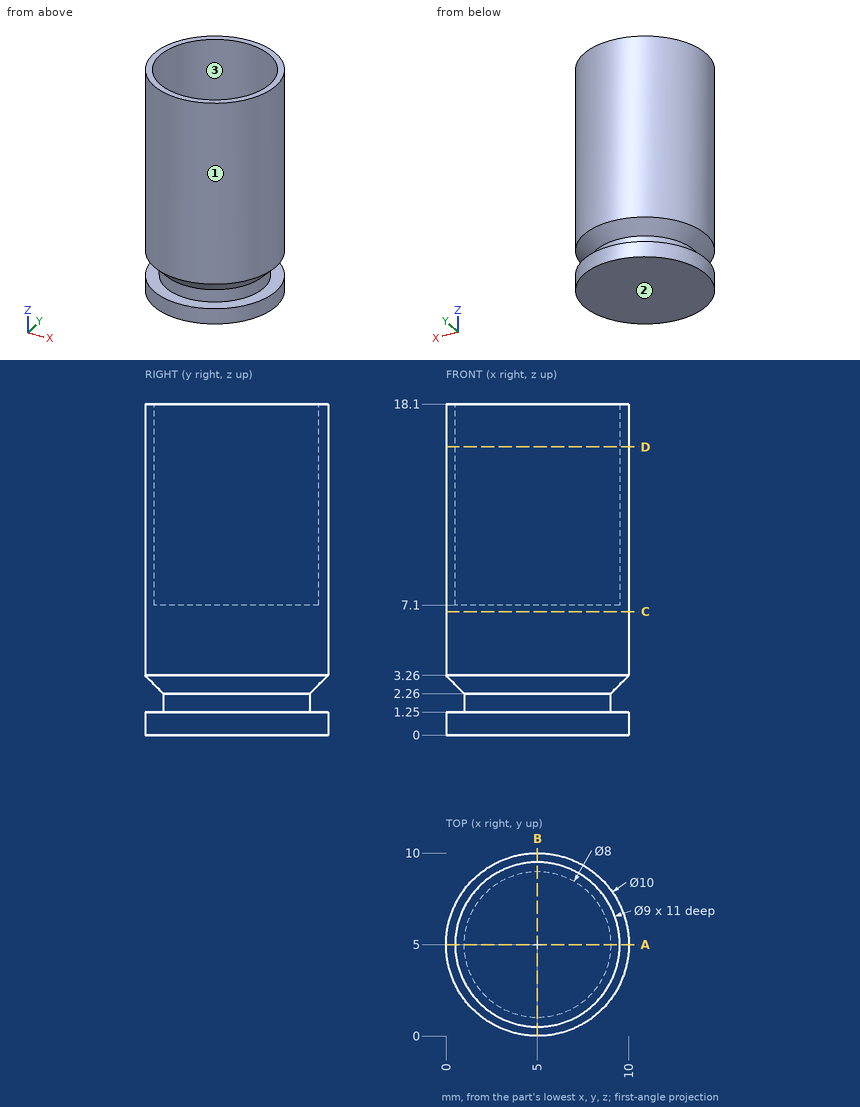
Can you work these out from the drawing? Everything is in mm from the part's minimum corner. Round coordinates to 2 decimals unless told otherwise and drop trailing zeros. Order: outer loops, then holes, each group sorted by start corner. A loop starts at its lowest first (then second) coordinate and runs counter-clockwise, first axis right, second up. Notation, with made-up numbers: M 47,-34 L 61,-34 A19 ccw 61,-29 Z; hole C 25,4 d6. An arc over 180 degrees is marked long. Answer as CSV lines item,"result".
Item 1: Imagine slicing it at C-C on z = 6.75. List the corners of the cut face in (x, y) for me.
From the geometry:
outline,"C 5,5 d10"
Item 2: Imagine slicing it at D-D on z = 15.75. List the corners of the cut face in (x, y) for me, and give its area (3 significant figures).
From the geometry:
outline,"C 5,5 d10; hole C 5,5 d9"
area,"14.9 mm2"
Item 3: We'd pull the mould along X, two halves only. Please class the marked faces 1, 2 and 3: +X half, -X half, draft (parallel to the pull), parting line (faces both ways), or undercut.
From the geometry:
face 1,"parting line"
face 2,"draft"
face 3,"undercut"
Item 4: Imagine slicing it at A-A on y = 5. List the corners of the cut face in (x, z) for me, and give its area (3 significant figures).
From the geometry:
outline,"M 0,0 L 10,0 L 10,1.25 L 9,1.25 L 9,2.26 L 10,3.26 L 10,18.1 L 9.5,18.1 L 9.5,7.1 L 0.5,7.1 L 0.5,18.1 L 0,18.1 L 0,3.26 L 1,2.26 L 1,1.25 L 0,1.25 Z"
area,"79.0 mm2"
Item 5: For pin 1 (1 mm diameter, centred on y = 2.5, z = 13, fed in from +X); pin 2 (2.5 mm diameter, centred on x = 3, y = 7, fed in from +Z); pin 3 (1.5 mm diameter, centred on x = 7.5, z = 8.5, fed in from +Y), each with a flat end and sliding along its axis, tell me the tip position at first contact or that it passes through.
From the geometry:
pin 1,"x = 9.58"
pin 2,"z = 7.1"
pin 3,"y = 9.68"
Item 6: Please list where these lines run through material, in increasing order: L1, parallel to Y at x = 5, z = 14; L2, parallel to Z at x = 1.25, y = 4.5; L3, parallel to Z at x = 3.25, y = 1.25. Write a range as [from, to].
From the geometry:
L1,"[0, 0.5], [9.5, 10]"
L2,"[0, 7.1]"
L3,"[0, 1.25], [2.4, 7.1]"
